Can you work these out from the model? Positions are in its coordinate system, mm. Give positions to 0.01 mm unless a question says otherwise; leave off trailing zeros. Write each loop counter-clockwise with the first axis right and the second up, starting at its lowest first coordinate (ties: lowest second). Pieces come first, ordered by that corner, then holes. Notation, with made-up numbers: (-37.75, 69) -> (-21.75, 69) arc R28 cw to (-21.75, 100) -> close; hole circle Ø7 at (-0.5, -4.5). An arc over 180 degrees is marked (long way). Answer as CSV lines item,"result". Start each with the question number.
1. If we section it at A-A on y = 9.25: Write out the boundary of the cut face in (x, z).
2. I need wall thicknesses on line 1 (X direction, y = 8.5, z = -32); line 2 (Z direction, x = 1, y = -1.75); line 3 (X direction, y = 4.5, z = -15). Which ranges of each line are inside material? Lowest first, please. Write a range as [from, to].
3. I'm going to push flat-ended pins straight in: P1, Ø5, axis at x = -10, y = 5.5, coming from the +Z side; P2, Ø12, axis at x = 14.5, y = 9, coming from the +Z side; P3, Ø1, axis at x = -16, z = -25.5, coming from the +Y side; P4, Ø1.8, axis at y = 6.5, z = -14, coming from the -X side. Where does each tip first touch, or does it pass through?
4. If we section it at C-C on x = -25: Write out the boundary of the cut face in (y, z) (3 decimals), plus the area to 3 significant figures.
5. If we section it at D-D on y = -1: Write out the boundary of the cut face in (x, z).
6. If we section it at B-B on z = -21: Write out the boundary of the cut face in (x, y) (3 decimals), plus the area to 3 significant figures.
```python
from build123d import *

# Parameters (mm, degrees)
BOSS_EXTRUDE1_DEPTH = 3.175
BOSS_EXTRUDE2_START = 17.78
BOSS_EXTRUDE2_DEPTH = 17.78
FILLET1_R           = 0.79375


with BuildPart() as part:
    # Sketch2 → Boss-Extrude1 (new body)
    with BuildSketch(Plane(origin=(0, 0, 0), x_dir=(1, 0, 0), z_dir=(0, 1, 0))):
        with BuildLine():
            ThreePointArc((0, 30.7975), (20.332846129, 24.964334619), (34.480947296, 9.239141982))
            Line((34.480947296, 9.239141982), (34.480947296, 15.906382448))
            ThreePointArc((34.480947296, 15.906382448), (32.596761403, 19.478189726), (30.343916909, 22.829705114))
            Line((30.343916909, 22.829705114), (39.484711098, 29.70691996))
            Line((39.484711098, 29.70691996), (29.497478634, 37.551994065))
            ThreePointArc((29.497478634, 37.551994065), (15.605618915, 45.130013985), (0, 47.752))
            Line((0, 47.752), (0, 30.7975))
        make_face()
    extrude(amount=-BOSS_EXTRUDE1_DEPTH)

    # Sketch2<3> → Boss-Extrude2 (add)
    with BuildSketch(Plane(origin=(0, 0, 0), x_dir=(1, 0, 0), z_dir=(0, 1, 0)).offset(BOSS_EXTRUDE2_START)):
        with BuildLine():
            Line((0, 37.973), (0, 30.7975))
            ThreePointArc((0, 30.7975), (20.332846129, 24.964334619), (34.480947296, 9.239141982))
            Line((34.480947296, 9.239141982), (34.480947296, 15.906382448))
            ThreePointArc((34.480947296, 15.906382448), (20.468703773, 31.984072518), (0, 37.973))
        make_face()
        with BuildLine():
            Line((0, 47.752), (0, 44.577))
            ThreePointArc((0, 44.577), (14.568011274, 42.129348162), (27.536210108, 35.055185949))
            Line((27.536210108, 35.055185949), (36.85939786, 27.731725813))
            Line((36.85939786, 27.731725813), (39.484711098, 29.70691996))
            Line((39.484711098, 29.70691996), (29.497478634, 37.551994065))
            ThreePointArc((29.497478634, 37.551994065), (15.605618915, 45.130013985), (0, 47.752))
        make_face()
    extrude(amount=-BOSS_EXTRUDE2_DEPTH)

    # Fillet1
    fillet1_edges = [part.edges().sort_by_distance(p)[0] for p in [
        (34.480947296, 7.3025, -9.239141982),
    ]]
    fillet(fillet1_edges, radius=FILLET1_R)

    # Mirror1: part across plane


with BuildPart() as part_1:
    add(part.part)
    add(part.part.mirror(Plane(origin=(0, -3.175, 0), x_dir=(0, 0, 1), z_dir=(1, 0, 0))))


solid = part_1.part
```
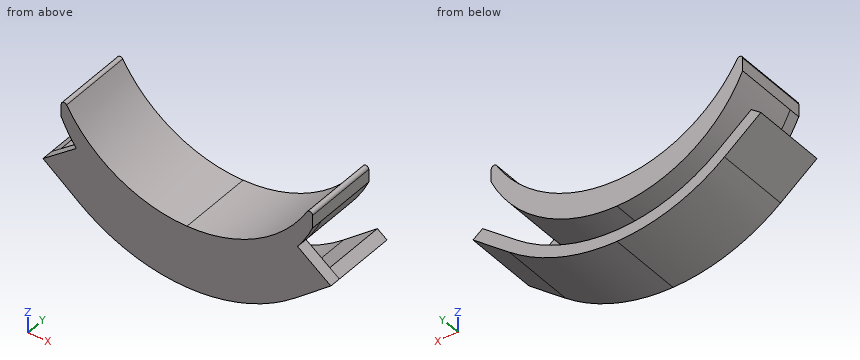
Computed values:
1,outline,"(-39.48, -29.71) -> (-29.5, -37.55) arc R47.75 ccw to (29.5, -37.55) -> (39.48, -29.71) -> (36.86, -27.73) -> (27.54, -35.06) arc R44.58 cw to (-27.54, -35.06) -> (-36.86, -27.73) -> close; (-34.48, -15.91) arc R37.97 ccw to (34.48, -15.91) -> (34.48, -12.39) arc R0.79 ccw to (33, -11.98) arc R38.35 cw to (-33, -11.98) arc R0.79 ccw to (-34.48, -12.39) -> close"
2,line 1,"x = [-36.57, -31.43], [-20.44, 20.44], [31.43, 36.57]"
2,line 2,"z = [-47.74, -30.78]"
2,line 3,"x = [-34.48, -31.02], [31.02, 34.48]"
3,P1,"stops at z = -28.7"
3,P2,"stops at z = -24.86"
3,P3,"passes through"
3,P4,"stops at x = -34.48"
4,outline,"(-3.175, -40.685) -> (17.78, -40.685) -> (17.78, -36.907) -> (0, -36.907) -> (0, -28.582) -> (17.78, -28.582) -> (17.78, -21.53) -> (-3.175, -21.53) -> close"
4,area,"253 mm2"
5,outline,"(-39.48, -29.71) -> (-29.5, -37.55) arc R47.75 ccw to (29.5, -37.55) -> (39.48, -29.71) -> (30.34, -22.83) arc R37.97 ccw to (34.48, -15.91) -> (34.48, -12.39) arc R0.79 ccw to (33, -11.98) arc R38.35 cw to (-33, -11.98) arc R0.79 ccw to (-34.48, -12.39) -> (-34.48, -15.91) arc R37.97 ccw to (-30.34, -22.83) -> close"
6,outline,"(-31.638, -3.175) -> (-25.604, -3.175) -> (-25.604, 17.78) -> (-31.638, 17.78) -> close; (25.604, -3.175) -> (31.638, -3.175) -> (31.638, 17.78) -> (25.604, 17.78) -> close"
6,area,"253 mm2"
